```python
from build123d import *

# Parameters (mm, degrees)
SKETCH1_R           = 9
BOSS_EXTRUDE1_DEPTH = 6


with BuildPart() as part:
    # Sketch1 → Boss-Extrude1 (new body)
    with BuildSketch(Plane.XY):
        with BuildLine():
            Line((3, 160), (37.5, 160))
            Line((37.5, 160), (37.5, 232.000025877))
            Line((37.5, 232.000025877), (17.5, 252.000025877))
            Line((17.5, 252.000025877), (-17.5, 252.000025877))
            Line((-17.5, 252.000025877), (-37.5, 232.000025877))
            Line((-37.5, 232.000025877), (-37.5, 160))
            Line((-37.5, 160), (-3, 160))
            Line((-3, 160), (-3, 198.5))
            ThreePointArc((-3, 198.5), (-4.060660172, 201.060660172), (-1.5, 200))
            Line((-1.5, 200), (1.5, 200))
            ThreePointArc((1.5, 200), (3, 201.5), (4.5, 200))
            ThreePointArc((4.5, 200), (4.060660172, 198.939339828), (3, 198.5))
            Line((3, 198.5), (3, 160))
        make_face()
        with Locations((9.65e-05, 239.99993797)):
            Circle(SKETCH1_R, mode=Mode.SUBTRACT)
    extrude(amount=BOSS_EXTRUDE1_DEPTH)


solid = part.part
```
Geometry: final body of the model. Coordinates: model frame, mm. A direction names the side the tool comes from. Coordinates: 2 decimals unless noted, no trailing zeros. Order: outer loops, then holes, each group sorted by start corner. A loop starts at its lowest first (then second) coordinate and runs counter-clockwise, first axis right, second up. Notation, with made-up numbers: (62, 9.25) - (108, 9.25) arc R23 ccw to (108, 21.25) - close; hole circle Ø1 at (39, 77). An arc over 180 degrees is marked (long way). Return JSON: item names as keys, results as strings. Group by question number.
1. Cut plane B-B (x = 7.5). Output: boundary loops of the cut face in (y, z).
2. Pin query (flat end, axial travel): pin 1 (1.5 mm diameter, centred on x = 0, z = 3, fed in from -Y); pin 2 (14.5 mm diameter, centred on x = 0, y = 240, fed in from +Z). Return the tip coordinate at first contact, or that it passes through.
3. Cut plane C-C (z = 4.55). Output: boundary loops of the cut face in (x, y), plus the area to 3 significant figures.
4. Pull-direction query (X, two-part tool) for faces 1 (the face through (-3, 179, 3)), 2 (the face through (3, 180, 3)), 3 (the face through (0, 252, 3)), 4 (the face through (27.6, 241.9, 3)); classes: pulls with the +X half, pulls with the -X half, needs draft (parallel to the pull), parting line crosses it, or undercut.
5. Set-up query: faces 5 (the face through (0, 200, 3)), 6 (the face through (37.5, 195, 3)). Return all of +Z, -Z, +X, -X, +Y, -Y with unobstructed straight access to the full face (end or side cutting, diameter ignored); none if empty.
6. Cut plane D-D (x = -23). Output: boundary loops of the cut face in (y, z), plus the area to 3 significant figures.
7. Material intervals for line 1 along X through (y, z) = (167.5, 4.4); line 2 along X through (y, z) = (234.5, 3.7); line 3 along Y through (x, z) = (5, 0.55), sorted ascending. Write a range as [from, to].
8. Cut plane A-A (y = 193.5). Output: boundary loops of the cut face in (x, z).
Resolved:
{
 "1": {"outline": "(160, 0) - (235.02, 0) - (235.02, 6) - (160, 6) - close; (244.98, 0) - (252, 0) - (252, 6) - (244.98, 6) - close"},
 "2": {"pin 1": "stops at y = 200", "pin 2": "passes through"},
 "3": {"outline": "(-37.5, 160) - (-3, 160) - (-3, 198.5) arc R1.5 cw (long way) to (-1.5, 200) - (1.5, 200) arc R1.5 cw (long way) to (3, 198.5) - (3, 160) - (37.5, 160) - (37.5, 232) - (17.5, 252) - (-17.5, 252) - (-37.5, 232) - close; hole circle Ø18 at (0, 240)", "area": "5,990 mm²"},
 "4": {"face 1": "undercut", "face 2": "undercut", "face 3": "needs draft", "face 4": "pulls with the +X half"},
 "5": {"face 5": "+Z, -Z, -Y", "face 6": "+Z, -Z, +X, +Y, -Y"},
 "6": {"outline": "(160, 0) - (246.5, 0) - (246.5, 6) - (160, 6) - close", "area": "519 mm²"},
 "7": {"line 1": "x = [-37.5, -3], [3, 37.5]", "line 2": "x = [-35, -7.12], [7.12, 35]", "line 3": "y = [160, 232.52], [247.48, 252]"},
 "8": {"outline": "(-37.5, 0) - (-3, 0) - (-3, 6) - (-37.5, 6) - close; (3, 0) - (37.5, 0) - (37.5, 6) - (3, 6) - close"}
}
